```python
from build123d import *

# Parameters (mm, degrees)
CUT_EXTRUDE1_DEPTH      = 44.589870827
CUT_EXTRUDE1_DEPTH_BACK = 44.589870827
SKETCH4_W               = 60
SKETCH4_H               = 60
BOSS_EXTRUDE1_DEPTH     = 4


with BuildPart() as part:
    # Sketch1 → Revolve1 (revolve)
    with BuildSketch(Plane.XY, mode=Mode.PRIVATE) as revolve1_sk:
        with BuildLine():
            Line((0, -23.350993377), (0, -27.350993377))
            ThreePointArc((0, -27.350993377), (18.81908657, -18.245354078), (23.358188619, 2.1621749))
            Line((23.358188619, 2.1621749), (19.462239628, 1.255657105))
            ThreePointArc((19.462239628, 1.255657105), (15.686507094, -15.757987178), (0, -23.350993377))
        make_face()
    revolve(revolve1_sk.sketch.rotate(Axis((0, 16.649006623, 0), (0, -1, 0)), 180), axis=Axis((0, 16.649006623, 0), (0, -1, 0)))

    # Sketch2 → Cut-Extrude1 (cut, two sides: drawn at the far end of the back side and taken through both)
    with BuildSketch(Plane.XY.offset(-CUT_EXTRUDE1_DEPTH_BACK)):
        with BuildLine():
            Line((0, 13.619569371), (-2, 13.619569371))
            Line((-2, 13.619569371), (-2, -6.380430629))
            ThreePointArc((-2, -6.380430629), (0, -8.380430629), (2, -6.380430629))
            Line((2, -6.380430629), (2, 13.619569371))
            Line((2, 13.619569371), (0, 13.619569371))
        make_face()
    extrude(amount=CUT_EXTRUDE1_DEPTH + CUT_EXTRUDE1_DEPTH_BACK, mode=Mode.SUBTRACT)

    # Sketch4 → Boss-Extrude1 (add)
    with BuildSketch(Plane(origin=(0, -27.350993377, 0), x_dir=(-1, 0, 0), z_dir=(0, -1, 0))):
        Rectangle(SKETCH4_W, SKETCH4_H)
    extrude(amount=-BOSS_EXTRUDE1_DEPTH)


solid = part.part
```
Model file for the job. Use its own axes, mm. A direction names the side the tool comes from. Coordinates: 2 decimals unless noted, no trailing zeros. Loops run counter-clockwise (first coordinate to the right, second up) from the corner with the lowest first, then second, coordinate; pieces in that order, holes last. Notation, with made-up numbers: (59, -13.5) - (86, -13.5) arc R30 cw to (86, 14.5) - close; hole circle Ø6 at (22.5, 76). An arc over 180 degrees is marked (long way). Write item = value, one per line. Start each with the question number.
Item 1: Wall check: probe 1 along Y at (x, z) = (-24.5, 22); probe 2 along Z at (x, y) = (-6, -10.75); probe 3 along Z at (x, y) = (-15, -14.5). Give the ranges that are in metal, low to high. Write a range as [from, to].
Item 2: 3-axis set-ups, long thin cutter, end or side, ignore diameter. For faces 4 (the face through (14, -23.351, 0)), 5 (the face through (0, -25, -30)), 6 (the face through (19.65, 1.3, -0.41)), 7 (the face through (-2, -2, 22)): which of +Z, -Z, +X, -X, +Y, -Y reach the whole face in a straight line?
Item 3: Drop flat-ended pins along their axis: pin 1 Ø8 at (x, y) = (20, -7) entering from -Z; pin 2 Ø5 at (y, z) = (-4, -22.5) entering from +X; pin 3 Ø1.4 at (y, z) = (-2, -22.5) entering from -X. Give the stop position or say it passes through.
Item 4: Saw through at D-D, the plane y = -10.25. List the corners of the cut face in (x, z).
Item 5: Saw through at C-C, the plane x = 0. List the corners of the cut face in (y, z), then the cut area to 3 significant figures.
Item 6: Pull direction X, two halves, no side cores. Call faces 1 (the face through (2, -2, 22)), 2 (the face through (-30, -25, 0)), 3 (the face through (0, -27.351, 0)): +X half, -X half, draft (parallel to the pull), parting line (faces both ways), or undercut.
Item 7: Saw through at B-B, the plane z = -25. List the corners of the cut face in (x, y), then the cut area to 3 significant figures.
Item 8: Saw through at A-A, the plane y = -4. List the corners of the cut face in (x, z), then the cut area to 3 significant figures.
Answers:
q1.probe_1 = [-27.35, -23.35]
q1.probe_2 = [-22.03, -17.59], [17.59, 22.03]
q1.probe_3 = [-15.06, -7.12], [7.12, 15.06]
q2.face_4 = none
q2.face_5 = -Z, +X, -X, +Y, -Y
q2.face_6 = +Y
q2.face_7 = +Z, -Z, +Y
q3.pin_1 = -17.59
q3.pin_2 = 13.25
q3.pin_3 = -9.95
q4.outline = circle Ø45.97 at (0, 0); hole circle Ø37.54 at (0, 0)
q5.outline = (-27.35, -30) - (-23.35, -30) - (-23.35, -13.27) arc R24 ccw to (-8.38, -23.47) - (-8.38, -19.36) arc R20 cw to (-8.38, 19.36) - (-8.38, 23.47) arc R24 ccw to (-23.35, 13.27) - (-23.35, 30) - (-27.35, 30) - close
q5.area = 404 mm2
q6.face_1 = undercut
q6.face_2 = -X half
q6.face_3 = draft
q7.outline = (-30, -27.35) - (30, -27.35) - (30, -23.35) - (-30, -23.35) - close
q7.area = 240 mm2
q8.outline = (-2, -23.91) - (-2, -19.89) arc R19.99 cw to (-2, 19.89) - (-2, 23.91) arc R23.99 ccw to start; (2, -23.91) arc R23.99 ccw to (2, 23.91) - (2, 19.89) arc R19.99 cw to (2, -19.89) - close
q8.area = 521 mm2
